Solid Edge part; units mm, degrees
sketch "Sketch1" plane through (0, 0, 0) normal (0, -1, 0) x (1, 0, 0)
  arc A0 (0, -40.3674) -> (0, 87.4202) centre (0, 23.5264) cw
  line L0 (0, 87.4202) -> (0, -40.3674)
revolve "RevolvedProtrusion1" add sketch "Sketch1" angle 360 about axis through (0, 0, 87.4202) along (0, 0, -1)
sketch "Sketch2" plane through (0, 0, 0) normal (0, -1, 0) x (1, 0, 0)
  line L0 (42.5325, 42.5325) -> (34.4095, 0)
  line L1 (0, -26.2866) -> (34.4095, 0)
extrude "Cutout1" cut sketch "Sketch2" along normal mid plane 225.678 material side at (38.5201, 0, 21.2569)
sketch "Sketch3" plane through (0, 0, 0) normal (0, -1, 0) x (1, 0, 0)
  line L0 (-34.4095, 42.5325) -> (0, 68.8191)
  line L1 (-42.5325, 0) -> (-34.4095, 42.5325)
extrude "ExtrudedCutout_2" cut sketch "Sketch3" along normal mid plane 171.0823 material side at (-17.2351, 0, 55.7155)
pattern_circular "Pattern1" count 5 over 360 about axis through (0, 0, 0) along (0, 0, 1) of "Cutout1", "ExtrudedCutout_2"
Can you work these out from the model? Positions are in its coordinate system, mm. Coordinates: 2 decimals unless noted, no trailing zeros. Loops run counter-clockwise (first coordinate to the right, second up) from the corner with the lowest first, then second, coordinate; pieces in that order, holes last.
Item 1: Please list where these lines run through material, in increasing order: L1, parallel to X at y = 11.5, z = 9; L2, parallel to Z at x = -4.5, y = -13.5; L3, parallel to Z at x = 22, y = -15.
Answers below:
L1: x = -36.3 to 36.13
L2: z = -17.44 to 57.95
L3: z = -9.48 to 48.49
Item 2: Suppose I cut it at A-A (y = -23.5). Please give me the cut outline in (x, z).
Answers below:
outline: (-34.9, 39.98) - (-25.46, 0) - (-7.64, -11.02) - (32.34, -1.58) - (34.41, 0) - (34.9, 2.55) - (25.46, 42.53) - (7.64, 53.55) - (-32.34, 44.11) - (-34.41, 42.53) - close
Item 3: Suppose I cut it at B-B (z = 40.5). Please give me the cut outline in (x, y), then the cut area to 3 significant figures.
Answers below:
outline: (-34.8, -23.81) - (-33.39, -25.74) - (11.89, -40.45) - (14.16, -39.71) - (42.14, -1.19) - (42.14, 1.19) - (14.16, 39.71) - (11.89, 40.45) - (-33.39, 25.74) - (-34.8, 23.81) - close
area: 4,390 mm2
Item 4: I'm going to push flat-ended pins straight in: pin 1 (8 mm diameter, centred on y = -22.5, z = 24, fed in from +X); pin 2 (1.5 mm diameter, centred on y = 0.5, z = 13.5, fed in from -X); pin 3 (6 mm diameter, centred on x = 30.5, y = -2, fed in from +Z). Where does each tip first touch, or does it pass through?
Answers below:
pin 1: stops at x = 33.62
pin 2: stops at x = -40.1
pin 3: stops at z = 51.36
Item 5: Suppose I cut it at D-D (y = 30). Please give me the cut outline in (x, z).
Answers below:
outline: (-27.53, 28.77) - (-20.74, 0) - (-9.75, -6.79) - (19.02, 0) - (27.53, 13.76) - (20.74, 42.53) - (9.75, 49.32) - (-19.02, 42.53) - close
Item 6: Suppose I cut it at C-C (x = 2). Please give me the cut outline in (y, z), then the cut area to 3 significant figures.
Answers below:
outline: (-40.45, 24.5) - (-35.53, 0) - (-1.45, -24.76) - (1.45, -24.76) - (35.53, 0) - (40.45, 24.5) - (36.83, 42.53) - (6.16, 64.82) - (0, 67.58) - (-6.16, 64.82) - (-36.83, 42.53) - close
area: 5,150 mm2
